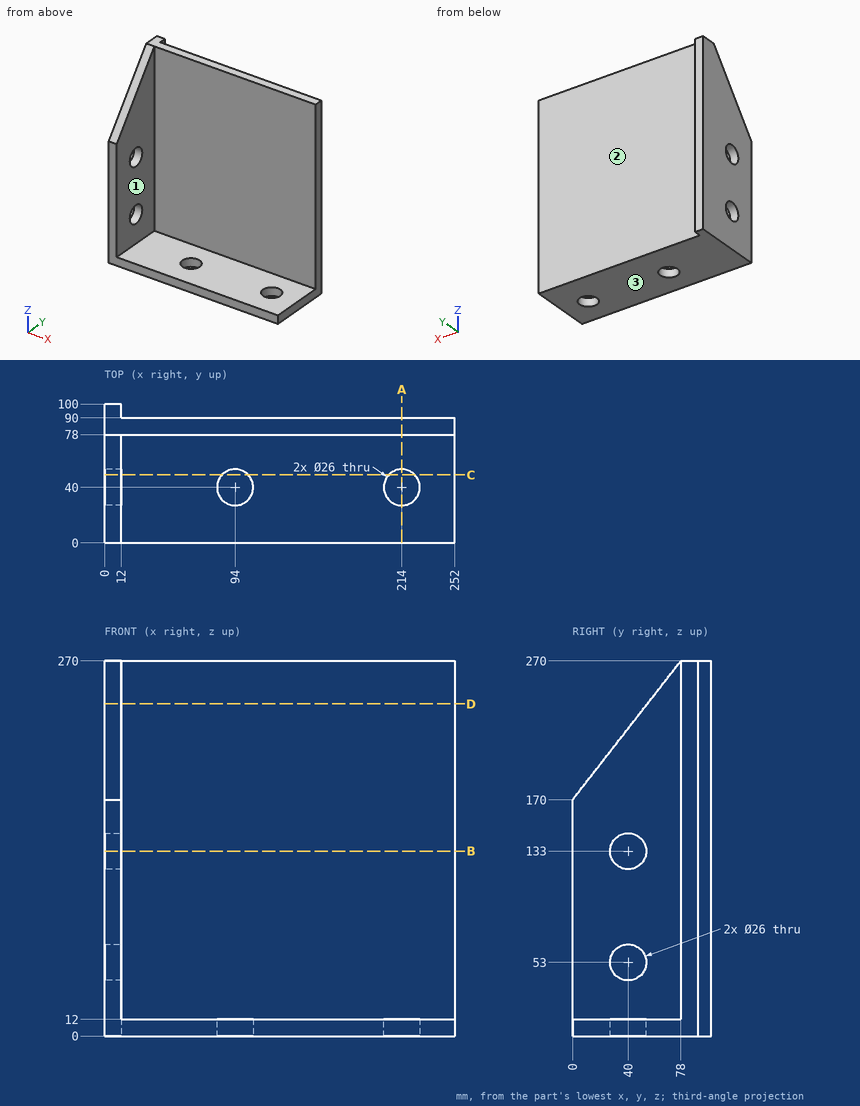
Could you check a few things on this drawing? It's one solid part, dimensions in mm from its lowest x, y, z. A direction names the side the tool comes from. Coordinates: 2 decimals unless noted, no trailing zeros. Order: outer loops, then holes, each group sorted by start corner. A loop starts at its lowest first (then second) coordinate and runs counter-clockwise, first axis right, second up. Notation, with made-up numbers: M -9,84 L 4,84 A8 ccw 4,94 Z; hole C -11,-12.5 d11. An arc over 180 degrees is marked long. Answer as a JSON object with one key per item and string values. Group by question number.
(1) Suppose I cut it at B-B, the plane z = 133. Please give me the cut outline in (x, y).
(2) I need wall thicknesses on probe 1 along Y at (x, z) = (5.5, 133); probe 2 along Y at (x, z) = (214, 7.25); probe 3 along X at (y, z) = (50, 70.5). Which ranges of each line are inside material? Lowest first, please.
(3) For pin 1 (8 mm diameter, centred on x = 52, z = 194, fed in from +Y); pin 2 (1 mm diameter, centred on x = 92, z = 156, fed in from -Y); pin 3 (2 mm diameter, centred on y = 30, z = 196.5, fed in from +X), each with a flat end and sliding along its axis, tell me the tip position at first contact or that it passes through.
(4) Suppose I cut it at C-C, the plane y = 49. Please give me the cut outline in (x, z), then the cut area to 3 significant figures.
(5) Which directions (+Z, -Z, +X, -X, +Y, -Y) give clear straight access to the entire face, cutting with the end or side of a thin tool? Please do the marked faces 1, 2 and 3.
(6) Suppose I cut it at D-D, the plane z = 239. Please give me the cut outline in (x, y).
(7) Suppose I cut it at A-A, the plane x = 214. Please give me the cut outline in (y, z), then the cut area to 3 significant figures.
Values found:
{
 "1": {"outline": "M 0,0 L 12,0 L 12,27 L 0,27 Z; M 0,53 L 12,53 L 12,78 L 252,78 L 252,90 L 12,90 L 12,100 L 0,100 Z"},
 "2": {"probe 1": "y = 0 to 27, 53 to 100", "probe 2": "y = 0 to 27, 53 to 90", "probe 3": "x = 0 to 12"},
 "3": {"pin 1": "stops at y = 90", "pin 2": "stops at y = 78", "pin 3": "stops at x = 12"},
 "4": {"outline": "M 0,0 L 84.62,0 L 84.62,12 L 12,12 L 12,43.62 L 0,43.62 Z; M 0,62.38 L 12,62.38 L 12,123.62 L 0,123.62 Z; M 0,142.38 L 12,142.38 L 12,232.82 L 0,232.82 Z; M 103.38,0 L 204.62,0 L 204.62,12 L 103.38,12 Z; M 223.38,0 L 252,0 L 252,12 L 223.38,12 Z", "area": "4,770 mm^2"},
 "5": {"face 1": "+Z, +X, -Y", "face 2": "+Z, -Z, +X, +Y", "face 3": "-Z, +X, -X, +Y, -Y"},
 "6": {"outline": "M 0,53.82 L 12,53.82 L 12,78 L 252,78 L 252,90 L 12,90 L 12,100 L 0,100 Z"},
 "7": {"outline": "M 0,0 L 27,0 L 27,12 L 0,12 Z; M 53,0 L 90,0 L 90,270 L 78,270 L 78,12 L 53,12 Z", "area": "3,860 mm^2"}
}
